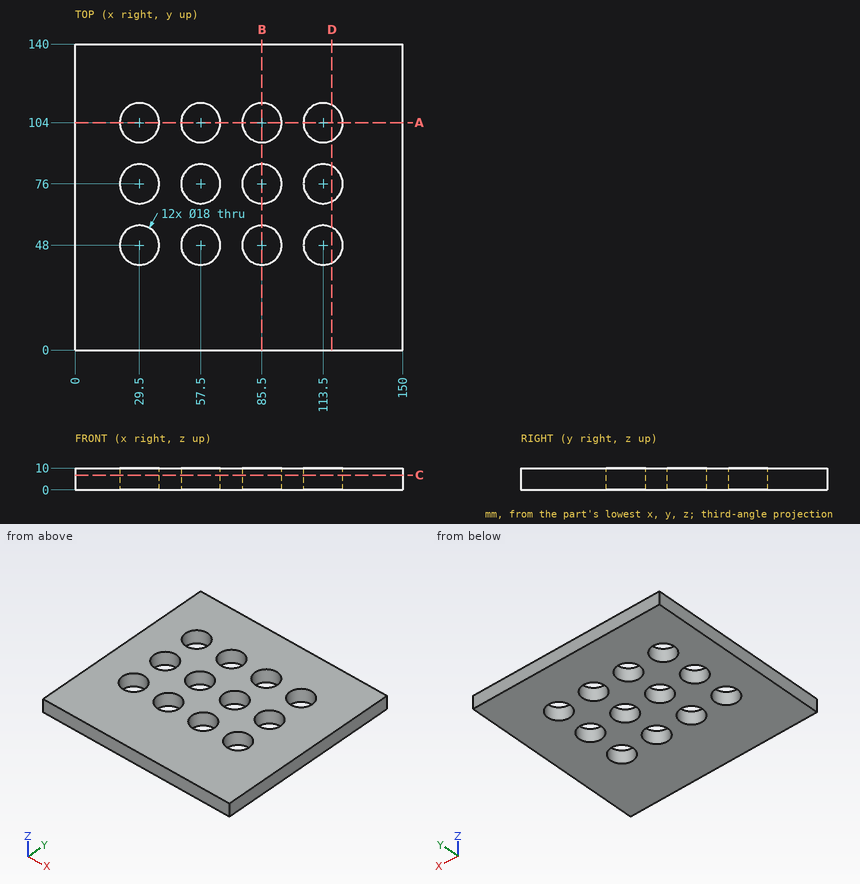
Verification items for this drawing (mm, ordinates from the low corner). Round coordinates to 2 decimals unless told otherwise and drop trailing zeros. Loops run counter-clockwise (first coordinate to the right, second up) from the corner with the lowest first, then second, coordinate; pieces in that order, holes last. Notation, with made-up numbers: M 81.5,19 L 120.5,19 A14 ccw 120.5,26 Z; hole C 84.5,24.25 d4. An arc over 180 degrees is marked long. Answer as a JSON object with one key per item and string values.
1. Gauge pin test, flat end, axial feed: P1, Ø14.5, axis at x = 29.5, y = 76, coming from the +Z side. Record the tip position at first contact, or that the pin passes through.
Reply:
{"P1": "passes through"}
2. Section check C-C (z = 6.75). State how many separate pieces and enclosed holes the cut face has, plus the area to 3 significant figures.
Reply:
{"separate pieces": "1", "enclosed holes": "12", "area": "17,900 mm²"}
3. Section check B-B (x = 85.5). Record the boundary of the cut face in (y, z), plus the area to 3 significant figures.
Reply:
{"outline": "M 0,0 L 39,0 L 39,10 L 0,10 Z; M 57,0 L 67,0 L 67,10 L 57,10 Z; M 85,0 L 95,0 L 95,10 L 85,10 Z; M 113,0 L 140,0 L 140,10 L 113,10 Z", "area": "860 mm²"}
4. Section check D-D (x = 117.5). Record the boundary of the cut face in (y, z), plus the area to 3 significant figures.
Reply:
{"outline": "M 0,0 L 39.94,0 L 39.94,10 L 0,10 Z; M 56.06,0 L 67.94,0 L 67.94,10 L 56.06,10 Z; M 84.06,0 L 95.94,0 L 95.94,10 L 84.06,10 Z; M 112.06,0 L 140,0 L 140,10 L 112.06,10 Z", "area": "916 mm²"}
5. Scan lines: line 1 (Y direction, x = 29.5, z = 5); line 2 (X direction, y = 104, z = 6.25); line 3 (Y direction, x = 24, z = 7.5). Record each from-to range of solid material in increasing order.
Reply:
{"line 1": "y = 0 to 39, 57 to 67, 85 to 95, 113 to 140", "line 2": "x = 0 to 20.5, 38.5 to 48.5, 66.5 to 76.5, 94.5 to 104.5, 122.5 to 150", "line 3": "y = 0 to 40.88, 55.12 to 68.88, 83.12 to 96.88, 111.12 to 140"}
6. Section check A-A (y = 104). Record the boundary of the cut face in (x, z), plus the area to 3 significant figures.
Reply:
{"outline": "M 0,0 L 20.5,0 L 20.5,10 L 0,10 Z; M 38.5,0 L 48.5,0 L 48.5,10 L 38.5,10 Z; M 66.5,0 L 76.5,0 L 76.5,10 L 66.5,10 Z; M 94.5,0 L 104.5,0 L 104.5,10 L 94.5,10 Z; M 122.5,0 L 150,0 L 150,10 L 122.5,10 Z", "area": "780 mm²"}
